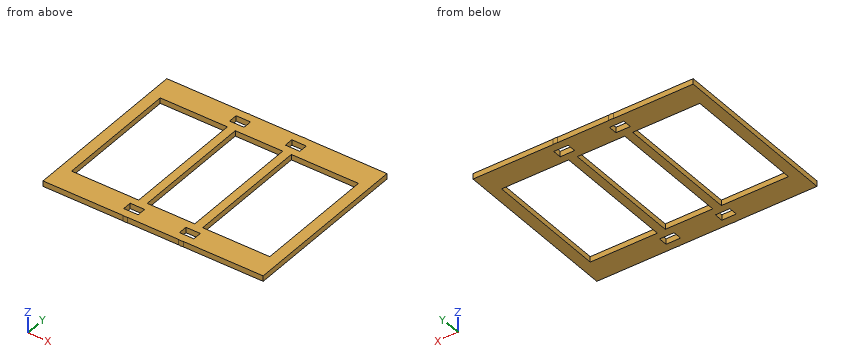
```python
from build123d import *

# Parameters (mm, degrees)
F0_W     = 10.5
F0_H     = 6.5
F0_W_2   = 17.25
F0_H_2   = 0.3298058208
F0_W_3   = 8
F0_H_3   = 17.6701941792
F0_H_4   = 44.5798058208
F1_DEPTH = 2


with BuildPart() as f1:
    # F0 (on Top) → F1 (new body, symmetric)
    with BuildSketch(Plane.XY):
        with BuildLine():
            Line((0, 62.25), (-18.4689140656, 62.25))
            ThreePointArc((-18.4689140656, 62.25), (-13.1608209467, 59.0737279689), (-11.0754554824, 53.25))
            ThreePointArc((-11.0754554824, 53.25), (-12.7768513778, 47.9279405512), (-17.25, 44.5798058208))
            Line((-17.25, 44.5798058208), (0, 44.5798058208))
            Line((0, 44.5798058208), (0, 62.25))
        make_face()
        with BuildLine():
            Line((-22.0310859344, 62.25), (-18.4689140656, 62.25))
            ThreePointArc((-18.4689140656, 62.25), (-20.25, 62.4245445176), (-22.0310859344, 62.25))
        make_face()
        with BuildLine():
            ThreePointArc((-11.0754554824, 53.25), (-13.1608209467, 59.0737279689), (-18.4689140656, 62.25))
            Line((-18.4689140656, 62.25), (-22.0310859344, 62.25))
            ThreePointArc((-22.0310859344, 62.25), (-29.4027939047, 53.8813721919), (-23.25, 44.5798058208))
            Line((-23.25, 44.5798058208), (-17.25, 44.5798058208))
            ThreePointArc((-17.25, 44.5798058208), (-12.7768513778, 47.9279405512), (-11.0754554824, 53.25))
        make_face()
        with Locations((-20.25, 53.25)):
            Rectangle(F0_W, F0_H, mode=Mode.SUBTRACT)
        with BuildLine():
            ThreePointArc((-23.25, 44.5798058208), (-29.4027939047, 53.8813721919), (-22.0310859344, 62.25))
            Line((-22.0310859344, 62.25), (-72, 62.25))
            Line((-72, 62.25), (-72, 44.5798058208))
            Line((-72, 44.5798058208), (-23.25, 44.5798058208))
        make_face()
        with Locations((-8.625, 44.4149029104)):
            Rectangle(F0_W_2, F0_H_2)
        with BuildLine():
            Line((-17.25, 44.25), (-17.25, 44.5798058208))
            ThreePointArc((-17.25, 44.5798058208), (-17.8537761691, 44.3939072691), (-18.4689140656, 44.25))
            Line((-18.4689140656, 44.25), (-17.25, 44.25))
        make_face()
        with BuildLine():
            ThreePointArc((-18.4689140656, 44.25), (-17.8537761691, 44.3939072691), (-17.25, 44.5798058208))
            Line((-17.25, 44.5798058208), (-23.25, 44.5798058208))
            ThreePointArc((-23.25, 44.5798058208), (-20.8813721919, 44.0972060953), (-18.4689140656, 44.25))
        make_face()
        with BuildLine():
            ThreePointArc((-18.4689140656, 44.25), (-20.8813721919, 44.0972060953), (-23.25, 44.5798058208))
            Line((-23.25, 44.5798058208), (-23.25, 0))
            Line((-23.25, 0), (-17.25, 0))
            Line((-17.25, 0), (-17.25, 44.25))
            Line((-17.25, 44.25), (-18.4689140656, 44.25))
        make_face()
        with Locations((-76, 53.4149029104)):
            Rectangle(F0_W_3, F0_H_3)
        with Locations((-76, 22.2899029104)):
            Rectangle(F0_W_3, F0_H_4)
    extrude(amount=F1_DEPTH, both=True)

    # F2: F1 across face


with BuildPart() as f1_1:
    add(f1.part)
    add(f1.part.mirror(Plane(origin=(0, 53.25, 0), x_dir=(0, 1, 0), z_dir=(1, 0, 0))))

    # F3: F1 across face


with BuildPart() as f1_2:
    add(f1_1.part)
    add(f1_1.part.mirror(Plane(origin=(-20.25, 0, 0), x_dir=(1, 0, 0), z_dir=(0, -1, 0))))


solid = f1_2.part
```
CAD build for the part. Positions are in the model's coordinates, mm. Round coordinates to 2 decimals unless told otherwise and drop trailing zeros. Write each loop counter-clockwise with the first axis right and the second up, starting at its lowest first coordinate (ties: lowest second). Pieces come first, ordered by that corner, then holes. Notation, with made-up numbers: M 2.25,-8.5 L 14.25,-8.5 A23 ccw 14.25,9.5 Z; hole C 58,-13.5 d9. An arc over 180 degrees is marked long. One line per question, with ' | ' between items.
1. Cut at A-A on x = -37.5. Write the cut outline in (y, z).
Working result:
outline: M -62.25,-2 L -44.58,-2 L -44.58,2 L -62.25,2 Z; M 44.58,-2 L 62.25,-2 L 62.25,2 L 44.58,2 Z
2. Probe L1, parallel to X at y = 28, z = 1.35; L2, parallel to X at y = 53, z = -1; L3, parallel to Y at x = -37.5, z = -1.55. List the from-to ranges inside material, lowest first. Write a range as from..to.
Working result:
L1: -80..-72, -23.25..-17.25, 17.25..23.25, 72..80 | L2: -80..-25.5, -15..15, 25.5..80 | L3: -62.25..-44.58, 44.58..62.25
3. Cut at B-B on y = 5.5. Write the cut outline in (x, z).
Working result:
outline: M -80,-2 L -72,-2 L -72,2 L -80,2 Z; M -23.25,-2 L -17.25,-2 L -17.25,2 L -23.25,2 Z; M 17.25,-2 L 23.25,-2 L 23.25,2 L 17.25,2 Z; M 72,-2 L 80,-2 L 80,2 L 72,2 Z
4. Cut at C-C on z = 0.8. Count the separate pieces of the cut face and the enclosed holes in it, and give its area (3 significant figures).
Working result:
separate pieces: 1 | enclosed holes: 7 | area: 7,900 mm2
5. Pin check, flat tips, straight feed: pin 1 Ø1.5 at (x, z) = (37.5, 1.5) entering from -Y; pin 2 Ø2 at (x, z) = (-3, 0) entering from +Y. Stop position of each tip, or through.
Working result:
pin 1: y = -62.25 | pin 2: y = 62.25
